from build123d import *

# Parameters (mm, degrees)
CROQUIS1_R              = 2.1
SALIENTE_EXTRUIR1_DEPTH = 250
MATRIZL1_COUNT          = 2
MATRIZL1_PITCH          = 20


with BuildPart() as part:
    # Croquis1 → Saliente-Extruir1 (new body)
    with BuildSketch(Plane.XY):
        Polygon((3, 8.2), (5.4, 8.2), (5.4, 6.85), (2.45, 3.9), (-2.55, 3.9), (-5.5, 6.85), (-5.5, 8.2), (-3, 8.2), (-4.8, 10), (-10, 10), (-10, 4.8), (-8.2, 3), (-8.2, 5.4), (-6.85, 5.4), (-3.9, 2.45), (-3.9, -2.55), (-6.85, -5.5), (-8.2, -5.5), (-8.2, -3), (-10, -4.8), (-10, -10), (-4.8, -10), (-3, -8.2), (-5.4, -8.2), (-5.4, -6.85), (-2.45, -3.9), (2.55, -3.9), (5.5, -6.85), (5.5, -8.2), (3, -8.2), (4.8, -10), (10, -10), (10, -4.8), (8.2, -3), (8.2, -5.4), (6.85, -5.4), (3.9, -2.45), (3.9, 2.55), (6.85, 5.5), (8.2, 5.5), (8.2, 3), (10, 4.8), (10, 10), (4.8, 10), align=None)
        Circle(CROQUIS1_R, mode=Mode.SUBTRACT)
    saliente_extruir1 = extrude(amount=SALIENTE_EXTRUIR1_DEPTH)

    # MatrizL1: Saliente-Extruir1 ×2
    with Locations(*[(0, -i * MATRIZL1_PITCH, 0) for i in range(1, MATRIZL1_COUNT)]):
        add(saliente_extruir1)


solid = part.part
Verification items for the finished model (mm, model axes). A direction names the side the tool comes from. Round coordinates to 2 decimals unless told otherwise and drop trailing zeros. Loops run counter-clockwise (first coordinate to the right, second up) from the corner with the lowest first, then second, coordinate; pieces in that order, holes last. Notation, with made-up numbers: (-16.75, -30) - (6.25, -30) arc R19 ccw to (6.25, -24) - close; hole circle Ø6 at (84, 86.5). An arc over 180 degrees is marked (long way). Answer in a Markdown table with one row per item. Add a question column.
Q1. Gauge pin test, flat ends, axial feed: pin 1 (1.5 mm diameter, centred on y = -23, z = 31.5, fed in from +X); pin 2 (2 mm diameter, centred on y = 4.5, z = 99, fed in from -X); pin 3 (5.5 mm diameter, centred on y = 0, z = 156.5, fed in from +X); pin 4 (5.5 mm diameter, centred on y = -19.5, z = 158.5, fed in from -X). Record the tip position at first contact, or that the pin passes through.
Q2. Section check B-B on y = 0. Enter the section's corners in (x, z), plus the area to 3 significant figures.
Q3. Tool access check on faces 5 (the face through (-5, -10, 250)), 6 (the face through (-3.9, 0, 123)), 7 (the face through (3.9, 0, 123)). Record the directions out of +Z, -Z, +X, -X, +Y, -Y that give a thin tool (end or side, any length) a straight path to the whole face; none if there is none.
Q4. Release check for a two-part mould opening along X. For faces 1 (the face through (0, -23.9, 123)), 2 (the face through (0, -16.1, 123)), 3 (the face through (-3.9, -20, 123)), 4 (the face through (7, -30, 123)) record: pulls with the +X half, pulls with the -X half, needs draft (parallel to the pull), parting line crosses it, or undercut.
Q5. Section check A-A on x = 0. Enter the section's corners in (y, z).
Q6. Material ranges on line 1 (Y direction, x = 0, z = 67); line 2 (Y direction, x = -7, z = 162.5); line 3 (X direction, y = -24, z = 227), recorded low to high.
Q7. Section check C-C on z = 209. State how many separate pieces and enclosed holes the cut face has, plus the area to 3 significant figures.
Found:
| question | item | result |
|---|---|---|
| 1 | pin 1 | stops at x = 8.95 |
| 1 | pin 2 | stops at x = -10 |
| 1 | pin 3 | stops at x = 4.2 |
| 1 | pin 4 | stops at x = -8.45 |
| 2 | outline | (-3.9, 0) - (-2.1, 0) - (-2.1, 250) - (-3.9, 250) - close; (2.1, 0) - (3.9, 0) - (3.9, 250) - (2.1, 250) - close |
| 2 | area | 900 mm² |
| 3 | face 5 | +Z, +X, -X, +Y, -Y |
| 3 | face 6 | +Z, -Z, -X |
| 3 | face 7 | +Z, -Z, +X |
| 4 | face 1 | undercut |
| 4 | face 2 | undercut |
| 4 | face 3 | pulls with the -X half |
| 4 | face 4 | needs draft |
| 5 | outline | (-23.9, 0) - (-22.1, 0) - (-22.1, 250) - (-23.9, 250) - close; (-17.9, 0) - (-16.1, 0) - (-16.1, 250) - (-17.9, 250) - close; (-3.9, 0) - (-2.1, 0) - (-2.1, 250) - (-3.9, 250) - close; (2.1, 0) - (3.9, 0) - (3.9, 250) - (2.1, 250) - close |
| 6 | line 1 | y = -23.9 to -22.1, -17.9 to -16.1, -3.9 to -2.1, 2.1 to 3.9 |
| 6 | line 2 | y = -30 to -25.5, -14.6 to -5.5, 5.4 to 10 |
| 6 | line 3 | x = -9.2 to -8.2, -5.35 to -2.55, 2.65 to 5.45, 8.2 to 9.2 |
| 7 | separate pieces | 1 |
| 7 | enclosed holes | 3 |
| 7 | area | 355 mm² |
